Read the model definition and answer for the solid it produces. Units are mm, in the model's axes. A direction names the side the tool comes from. Give positions to 0.01 mm unless a question says otherwise; leave off trailing zeros. Order: outer loops, then holes, each group sorted by start corner. A loop starts at its lowest first (then second) coordinate and runs counter-clockwise, first axis right, second up. Notation, with made-up numbers: (-29.75, -29.5) - (19.25, -29.5) arc R10 ccw to (19.25, -18.5) - close; hole circle Ø8 at (-35, 36.5). An arc over 180 degrees is marked (long way). Write each question's results on one line, items separated by ' | '.
from build123d import *

# Parameters (mm, degrees)
FILLET1_R = 4.7625


with BuildPart() as part:
    # Sketch1 → Revolve1 (revolve)
    with BuildSketch(Plane.XY, mode=Mode.PRIVATE) as revolve1_sk:
        Polygon((0, 11.1125), (12.7, 11.1125), (14.007022457, 18.524992696), (39.159831403, 22.059989461), (39.159831403, 20.456888189), (15.594522457, 17.145), (14.530829946, 11.1125), (25.4, 11.1125), (25.4, 9.525), (0, 9.525), align=None)
    revolve(revolve1_sk.sketch.rotate(Axis((0, 0, 0), (1, 0, 0)), 90), axis=Axis((0, 0, 0), (1, 0, 0)))

    # Fillet1
    fillet1_edges = [part.edges().sort_by_distance(p)[0] for p in [
        (14.007022457, 0, -18.524992696),
        (15.594522457, 0, -17.145),
    ]]
    fillet(fillet1_edges, radius=FILLET1_R)


solid = part.part
(1) For faces 1 (the face through (20, -7.5, -8.2)), 2 (the face through (26.035, 7.743, 18.674)), determine the directions among +Z, -Z, +X, -X, +Y, -Y from which every point of the face is accessible in a straight line to the end or side of a thin tool.
Conclusion:
face 1: +X | face 2: -X
(2) The mould has two halves that part along Y. Classify faces 3 (the face through (0, -8.3, 5)), 4 (the face through (12.52, 9.3, -2.06)), 5 (the face through (26.71, 18.26, -4.06)), 6 (the face through (6.4, -7.5, -8.2)): pulls with the +Y half, pulls with the -Y half, needs draft (parallel to the pull), parting line crosses it, or undercut.
Conclusion:
face 3: needs draft | face 4: undercut | face 5: undercut | face 6: parting line crosses it
(3) Consider probe 1 along Y at (x, z) = (7, 0) (1 decimal); probe 2 along Y at (x, z) = (24.5, 7.5); probe 3 along Y at (x, z) = (16, 8.5). Determine where each line is inside the solid, lowest interval first. Write a range as [from, to].
Conclusion:
probe 1: [-11.1, -9.5], [9.5, 11.1] | probe 2: [-18.54, -16.8], [-8.2, -5.87], [5.87, 8.2], [16.8, 18.54] | probe 3: [-16.51, -13.47], [-7.16, -4.3], [4.3, 7.16], [13.47, 16.51]
(4) Each of these flat-tipped pins is pushed along its axis until it touches: pin 1 (3 mm diameter, centred on y = -11, z = -5, fed in from -X); pin 2 (4 mm diameter, centred on x = 34, y = 16, fed in from -Z); pin 3 (5 mm diameter, centred on y = 7.5, z = 12, fed in from +X); pin 4 (5 mm diameter, centred on x = 7, z = 8, fed in from +Y). Where does it stop, or does it pass through?
Conclusion:
pin 1: x = 0 | pin 2: z = -16.14 | pin 3: x = 16.74 | pin 4: y = 9.66
(5) Section B-B (x = 36.5) is taken. Give the vertices of the cut face in (y, z).
Conclusion:
outline: circle Ø43.37 at (0, 0); hole circle Ø40.17 at (0, 0)
